Input: part model. Units: mm. Frame: model coordinates. Coordinates: 2 decimals unless noted, no trailing zeros. Write each loop counter-clockwise with the first axis right and the second up, starting at its lowest first coordinate (ties: lowest second). Pieces come first, ordered by that corner, then holes. Notation, with made-up numbers: (21.5, -32.75) - (61.5, -32.75) arc R28 ccw to (61.5, 3.25) - close; hole circle Ø1 at (28, -33). An arc over 180 degrees is marked (long way). Put each result on its own line as item: value. Start each with the question number.
1. Cut plane B-B, the plane y = 34. Return loops of the section in (x, z), and give its area (3 significant figures).
2. Line query: line 1 (Y direction, x = 4, z = 0.6); line 2 (Y direction, x = 29.7, z = 1.4); line 3 (X direction, y = 34, z = 0.65). Output: solid intervals per line, ascending.
3. Pull-direction query (Y, two-part tool) for faces 1 (the cylindrical face through (4, 33, 1)), 2 (the cylindrical face through (88.95, 37.5, 0.99)), 3 (the flat face through (0, 19, 1)), 4 (the cylindrical face through (89, 1.05, 0.99)); classes: released by +Y, released by -Y, zero draft, split by the parting line, or undercut.
4. Cut plane A-A, the plane z = 0.3. Count the separate pieces of the cut face and the enclosed holes in it, and give its area (3 significant figures).
5. Cut plane C-C, the plane x = 19.5. Return loops of the section in (y, z).
Autodesk Fusion 360 part; units mm, degrees
sketch "スケッチ1" plane through (0, 0, 0) normal (0, 0, 1) x (1, 0, 0)
  line L0 (3.5, 0) -> (86.5, 0)
  line L1 (90, 3.5) -> (90, 35)
  line L2 (86.5, 38.5) -> (3.5, 38.5)
  line L3 (0, 35) -> (0, 3.5)
  line L4 (0, 19.25) -> (90, 19.25)
  arc A0 (3.5, 38.5) -> (0, 35) centre (3.5, 35) ccw
  arc A1 (90, 35) -> (86.5, 38.5) centre (86.5, 35) ccw
  arc A2 (86.5, 0) -> (90, 3.5) centre (86.5, 3.5) ccw
  arc A3 (0, 3.5) -> (3.5, 0) centre (3.5, 3.5) ccw
  point P0 (90, 0)
  point P1 (0, 38.5)
  dimension "d1" = 90
  dimension "d2" = 38.5
  dimension "d3" = 3.5
extrude "押し出し1" add sketch "スケッチ1" along normal blind 2
sketch "スケッチ2" plane through (0, 0, 2) normal (0, 0, 1) x (-1, 0, 0)
  arc A0 (0, -3.5) -> (-3.5, 0) centre (-3.5, -3.5) ccw
  line L0 (-3.5, 0) -> (-86.5, 0)
  arc A1 (-86.5, 0) -> (-90, -3.5) centre (-86.5, -3.5) ccw
  line L1 (-90, -3.5) -> (-90, -35)
  arc A2 (-90, -35) -> (-86.5, -38.5) centre (-86.5, -35) ccw
  line L2 (-86.5, -38.5) -> (-3.5, -38.5)
  arc A3 (-3.5, -38.5) -> (0, -35) centre (-3.5, -35) ccw
  line L3 (0, -35) -> (0, -3.5)
  line L4 (-45, -38.5) -> (-45, 0)
  line L5 (0, -19.25) -> (-90, -19.25)
  line L6 (-45, -19.25) -> (-50.1, -19.25)
  line L7 (-50.1, -19.25) -> (-60.3, -19.25)
  line L8 (-60.3, -19.25) -> (-70.5, -19.25)
  point P0 (-50.1, -19.25)
  point P1 (-60.3, -19.25)
  point P2 (-70.5, -19.25)
  point P3 (-39.9, -19.25)
  point P4 (-29.7, -19.25)
  point P5 (-19.5, -19.25)
  dimension "d6" = 5.1
  dimension "d7" = 10.2
  dimension "d8" = 10.2
hole "穴1" at (19.5, 19.25, 2) at (29.7, 19.25, 2) at (39.9, 19.25, 2) at (50.1, 19.25, 2) at (60.3, 19.25, 2) at (70.5, 19.25, 2) direction (0, 0, -1) diameter 5.1 depth 2 tip angle 180
sketch "スケッチ3" plane through (0, 0, 2) normal (0, 0, 1) x (-1, 0, 0)
  circle A0 centre (-60.3, -19.25) radius 2.55
  circle A1 centre (-39.9, -19.25) radius 2.55
  circle A2 centre (-19.5, -19.25) radius 2.55
  circle A3 centre (-29.7, -19.25) radius 2.55
  circle A4 centre (-50.1, -19.25) radius 2.55
  circle A5 centre (-70.5, -19.25) radius 2.55
  arc A6 (0, -3.5) -> (-3.5, 0) centre (-3.5, -3.5) ccw
  line L0 (-3.5, 0) -> (-86.5, 0)
  arc A7 (-86.5, 0) -> (-90, -3.5) centre (-86.5, -3.5) ccw
  line L1 (-90, -3.5) -> (-90, -35)
  arc A8 (-90, -35) -> (-86.5, -38.5) centre (-86.5, -35) ccw
  line L2 (-86.5, -38.5) -> (-3.5, -38.5)
  arc A9 (-3.5, -38.5) -> (0, -35) centre (-3.5, -35) ccw
  line L3 (0, -35) -> (0, -3.5)
  line L4 (-4, -4) -> (-4, -34)
hole "穴2" at (4, 4, 2) at (4, 34, 2) direction (0, 0, -1) diameter 2 depth 2 tip angle 180
sketch "スケッチ5" plane through (0, 0, 0) normal (0, 0, 1) x (1, 0, 0)
sketch "スケッチ6" plane through (0, 0, 0) normal (0, 0, 1) x (1, 0, 0)
Report:
1. outline: (0, 0) - (3, 0) - (3, 2) - (0, 2) - close; (5, 0) - (90, 0) - (90, 2) - (5, 2) - close
1. area: 176 mm^2
2. line 1: y = 0 to 3, 5 to 33, 35 to 38.5
2. line 2: y = 0 to 16.7, 21.8 to 38.5
2. line 3: x = 0 to 3, 5 to 90
3. face 1: undercut
3. face 2: released by +Y
3. face 3: zero draft
3. face 4: released by -Y
4. separate pieces: 1
4. enclosed holes: 8
4. area: 3,330 mm^2
5. outline: (0, 0) - (16.7, 0) - (16.7, 2) - (0, 2) - close; (21.8, 0) - (38.5, 0) - (38.5, 2) - (21.8, 2) - close
